from build123d import *

# Parameters (mm, degrees)
SKETCH1_R           = 66.04
BOSS_EXTRUDE1_DEPTH = 6.35
SKETCH2_R           = 31.877
CUT_EXTRUDE1_DEPTH  = 6.35
SKETCH3_R           = 5
CUT_EXTRUDE2_DEPTH  = 6.35


with BuildPart() as part:
    # Sketch1 → Boss-Extrude1 (new body)
    with BuildSketch(Plane(origin=(0, 0, 0), x_dir=(1, 0, 0), z_dir=(0, 1, 0))):
        with Locations(Location((0, 0, 0), (0, 0, 270))):
            Circle(SKETCH1_R)
    extrude(amount=BOSS_EXTRUDE1_DEPTH)

    # Sketch2 → Cut-Extrude1 (cut)
    with BuildSketch(Plane(origin=(0, 6.35, 0), x_dir=(1, 0, 0), z_dir=(0, 1, 0))):
        with Locations(Location((0, 0, 0), (0, 0, 270))):
            Circle(SKETCH2_R)
    extrude(amount=-CUT_EXTRUDE1_DEPTH, mode=Mode.SUBTRACT)

    # Sketch3 → Cut-Extrude2 (cut)
    with BuildSketch(Plane(origin=(0, 6.35, 0), x_dir=(1, 0, 0), z_dir=(0, 1, 0))):
        with Locations(Location((38.1, -10.16, 0), (0, 0, 270))):
            Circle(SKETCH3_R)
        with Locations(Location((-38.1, -10.16, 0), (0, 0, 270))):
            Circle(SKETCH3_R)
    extrude(amount=-CUT_EXTRUDE2_DEPTH, mode=Mode.SUBTRACT)


solid = part.part
CAD build for the part. Positions are in the model's coordinates, mm. Give positions to 0.01 mm unless a question says otherwise; leave off trailing zeros. Loops run counter-clockwise (first coordinate to the right, second up) from the corner with the lowest first, then second, coordinate; pieces in that order, holes last. Notation, with made-up numbers: M 11,56 L 52,56 A8 cw 52,63 Z; hole C 72,56 d6. An arc over 180 degrees is marked long. Answer in a Markdown table with one row per item. Add a question column.
Item 1: Band-saw the part on B-B on x = 38.1. Give the cut face in (y, z), then the cut area to 3 significant figures.
Item 2: Band-saw the part on D-D on z = 53.5. Give the cut face in (x, y).
Item 3: Drop flat-ended pins along their axis: P1, Ø3, axis at x = -45.5, z = -11.5, coming from the -Y side; P2, Ø1.5, axis at y = 3, z = 24, coming from the -X side; P3, Ø1, axis at y = 1, z = -27, coming from the +X side; P4, Ø2, axis at y = 0.5, z = -31, coming from the -X side. Give the stop position or say it passes through.
Item 4: Probe probe 1 along X at (y, z) = (4.25, 10.16); probe 2 along X at (y, z) = (2, 8); probe 3 along Z at (x, y) = (-1, 0.5). List the from-to ranges inside material, lowest first.
Item 5: Band-saw the part on A-A on z = 0. Give the cut face in (x, y), then the cut area to 3 significant figures.
Item 6: Band-saw the part on C-C on y = 2.25. Give the cut face in (x, z).
Item 7: Mould opens along Z. For faces 1 (the face through (-28, 0, -16)), 2 (the face through (-40.18, 3.13, -52.41)), 3 (the face through (31.606, 3.219, -4.15)) say: +Z half, -Z half, draft (parallel to the pull), parting line (faces both ways), or undercut.
Reply:
| question | item | result |
|---|---|---|
| 1 | outline | M 0,-53.94 L 6.35,-53.94 L 6.35,5.16 L 0,5.16 Z; M 0,15.16 L 6.35,15.16 L 6.35,53.94 L 0,53.94 Z |
| 1 | area | 622 mm^2 |
| 2 | outline | M -38.72,0 L 38.72,0 L 38.72,6.35 L -38.72,6.35 Z |
| 3 | P1 | stops at y = 0 |
| 3 | P2 | stops at x = -61.81 |
| 3 | P3 | stops at x = 60.49 |
| 3 | P4 | stops at x = -58.83 |
| 4 | probe 1 | x = -65.25 to -43.1, -33.1 to -30.21, 30.21 to 33.1, 43.1 to 65.25 |
| 4 | probe 2 | x = -65.55 to -42.61, -33.59 to -30.86, 30.86 to 33.59, 42.61 to 65.55 |
| 4 | probe 3 | z = -66.03 to -31.86, 31.86 to 66.03 |
| 5 | outline | M -66.04,0 L -31.88,0 L -31.88,6.35 L -66.04,6.35 Z; M 31.88,0 L 66.04,0 L 66.04,6.35 L 31.88,6.35 Z |
| 5 | area | 434 mm^2 |
| 6 | outline | C 0,0 d132.08; hole C -38.1,10.16 d10; hole C 0,0 d63.75; hole C 38.1,10.16 d10 |
| 7 | face 1 | draft |
| 7 | face 2 | parting line |
| 7 | face 3 | undercut |
